```python
from build123d import *

# Parameters (mm, degrees)
F0_W     = 150
F0_H     = 250
F1_DEPTH = 100
F2_T     = -2.5
F3_R     = 5
F4_DEPTH = 200


with BuildPart() as f1:
    # F0 (on Top) → F1 (new body)
    with BuildSketch(Plane.XY):
        with Locations((0, -125)):
            Rectangle(F0_W, F0_H)
    extrude(amount=F1_DEPTH)

    # F2
    f2_openings = [f1.faces().sort_by_distance(p)[0] for p in [
        (0, -125, 0),
    ]]
    offset(amount=F2_T, openings=f2_openings)

    # F3 (on face) → F4 (join)
    with BuildSketch(Plane.XY.offset(100)):
        with Locations((0, -20.85017)):
            Circle(F3_R)
    extrude(amount=F4_DEPTH)


solid = f1.part
```
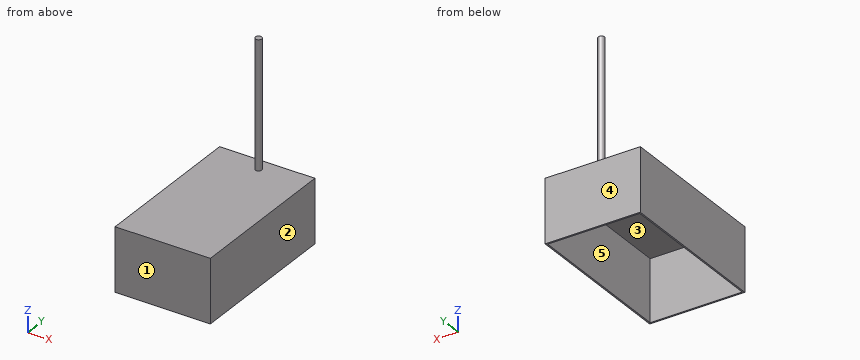
Verification items for the finished model (mm, model axes). Face numbers are marked on the shaded views. A direction names the side the tool comes from. Coordinates: 2 decimals unless noted, no trailing zeros. Write each loop counter-clockwise with the first axis right and the second up, starting at its lowest first coordinate (ties: lowest second). Pieces come first, ordered by that corner, then holes. Notation, with made-up numbers: (-34, -39.5) - (-22, -39.5) arc R29 ccw to (-22, -4.5) - close; hole circle Ø10 at (28, 40). An arc over 180 degrees is marked (long way). Write item = value, one per line.
Q1. Mould release check, pull along Y, two halves, no side actions. Record for the marked faces 1, 2 and 3: released by +Y, released by -Y, zero draft, split by the parting line, or undercut.
Answer:
face_1 = released by -Y
face_2 = zero draft
face_3 = undercut
Q2. Cross-section at B-B (y = -211.5). Enter the section's corners in (x, z), plus the area to 4 significant figures.
Answer:
outline = (-75, 0) - (-72.5, 0) - (-72.5, 97.5) - (72.5, 97.5) - (72.5, 0) - (75, 0) - (75, 100) - (-75, 100) - close
area = 862.5 mm²
Q3. Cross-section at A-A (z = 77.5). Enter the section's corners in (x, y).
Answer:
outline = (-75, -250) - (75, -250) - (75, 0) - (-75, 0) - close; hole (-72.5, -247.5) - (72.5, -247.5) - (72.5, -2.5) - (-72.5, -2.5) - close
Q4. Material ranges on L1, parallel to X at y = -177, z = 37; L2, parallel to Y at x = -49, z = 26; L3, parallel to Z at x = 31, y = -123, recorded low to high. Write a range as from..to.
Answer:
L1 = -75..-72.5, 72.5..75
L2 = -250..-247.5, -2.5..0
L3 = 97.5..100
Q5. Cross-section at C-C (x = 64). Enter the section's corners in (y, z), plus the area to 3 significant figures.
Answer:
outline = (-250, 0) - (-247.5, 0) - (-247.5, 97.5) - (-2.5, 97.5) - (-2.5, 0) - (0, 0) - (0, 100) - (-250, 100) - close
area = 1,110 mm²
Q6. Go/stop test with flat-tipped pins: pin 1 Ø4 at (x, y) = (-21, -174.5) entering from +Z; pin 2 Ø8 at (x, y) = (-49, -118) entering from -Z. Record where each tip stops, or that it passes through.
Answer:
pin_1 = 100
pin_2 = 97.5
Q7. Access from +Z, -Z, +X, -X, +Y, -Y to the whole of each face (thin tool, end or side, straight path). Record for the marked faces 4 and 5.
Answer:
face_4 = +Z, -Z, +X, -X, +Y
face_5 = -Z
Q8. Cross-section at D-D (x = 0). Enter the section's corners in (y, z), plus the area to 3 significant figures.
Answer:
outline = (-250, 0) - (-247.5, 0) - (-247.5, 97.5) - (-2.5, 97.5) - (-2.5, 0) - (0, 0) - (0, 100) - (-15.85, 100) - (-15.85, 300) - (-25.85, 300) - (-25.85, 100) - (-250, 100) - close
area = 3,110 mm²
